from build123d import *

# Parameters (mm, degrees)
F0_W     = 50.0364415348
F0_H     = 37.788476795
F1_DEPTH = 81.28
F2_R     = 5.08
F3_T     = -2.54


# Not quite as in the source:
# - a shell that OpenCascade refuses in one call is made with other operations: the cavity is built on its own and cut out


with BuildPart() as f1:
    # F0 (on Front) → F1 (new body)
    with BuildSketch(Plane.XZ):
        with Locations((25.0182207674, -18.8942383975)):
            Rectangle(F0_W, F0_H)
    extrude(amount=F1_DEPTH)

    # F2
    f2_edges = [f1.edges().sort_by_distance(p)[0] for p in [
        (25.018221, -81.28, 0),
        (0, -81.28, -18.894238),
        (25.018221, -81.28, -37.788477),
        (50.036442, -81.28, -18.894238),
    ]]
    fillet(f2_edges, radius=F2_R)

    # F3: a shell. OpenCascade refuses it in one call, so the cavity is built on its own and cut out:
    # the body offset inwards by the wall thickness, plus a prism from it out through each open face.
    f3_core = offset(f1.part, amount=F3_T, mode=Mode.PRIVATE)
    f3_exits = [f3_core.faces().sort_by_distance(p)[0] for p in [
        (25.018221, -78.74, -18.894238),
    ]]
    add(f3_core, mode=Mode.SUBTRACT)
    extrude(f3_exits, amount=-F3_T, mode=Mode.SUBTRACT)


solid = f1.part
Could you check a few things on this model? Use its own coordinates, in mm. A direction names the side the tool comes from. Give positions to 0.01 mm unless a question says otherwise; leave off trailing zeros. Order: outer loops, then holes, each group sorted by start corner. A loop starts at its lowest first (then second) coordinate and runs counter-clockwise, first axis right, second up. Notation, with made-up numbers: (51, 10.25) - (66, 10.25) arc R6 ccw to (66, 16.25) - close; hole circle Ø9 at (51, 76). An arc over 180 degrees is marked (long way). Return JSON: item names as keys, results as strings. Group by question number.
Q1. Thinking about a two-plate mould opening in X: for faces 1 (the face through (25.37, -79.75, -36.34)), 2 (the face through (25.3, -78, -34.5)), 3 (the face through (25.333, -77.976, -3.264)), 4 (the face through (0, -38, -19)), which applies, pulls with the +X half, pulls with the -X half, needs draft (parallel to the pull), parting line crosses it, or undercut?
Q2. Which directions (+Z, -Z, +X, -X, +Y, -Y) give clear straight access to the entire face, cutting with the end or side of a thin tool? Please do faces 5 (the face through (25, -39, -2.54)), 6 (the face through (25, -80, -5.08)), 7 (the face through (25, -38, 0)).
Q3. Please list where these lines run through material, in increasing order: line 1 along X through (y, z) = (-54, -7.5); line 2 along Z through (x, y) = (16, -9.5); line 3 along Y through (x, z) = (4, -20). Write a range as [from, to].
Q4. Suppose I cut it at B-B, the plane z = -29. Please give me the cut outline in (x, y), and give its area (3 significant figures).
Q5. Will these pins go through, and if not, where does the flat tip stop? pin 1 Ø1.5 at (x, z) = (11.5, -20) entering from +Y; pin 2 Ø0.8 at (x, y) = (31, -79.5) entering from +Z; pin 3 Ø0.8 at (x, y) = (20.5, -80.5) entering from -Z; pin 4 Ø4 at (x, z) = (18, -15.5) entering from -Y.
Q6. Suppose I cut it at A-A, the plane y = -55.5. Please give me the cut outline in (x, z).
Q7. Suppose I cut it at C-C, the plane x = 12. Please give me the cut outline in (y, z), and give its area (3 significant figures).
Resolved:
{
 "1": {"face 1": "needs draft", "face 2": "undercut", "face 3": "undercut", "face 4": "pulls with the -X half"},
 "2": {"face 5": "none", "face 6": "-Y", "face 7": "+Z, +X, -X, +Y, -Y"},
 "3": {"line 1": "x = [0, 2.54], [47.5, 50.04]", "line 2": "z = [-37.79, -35.25], [-2.54, 0]", "line 3": "y = [-81.16, -78.5], [-2.54, 0]"},
 "4": {"outline": "(0, -76.2) arc R5.08 ccw to (5.08, -81.28) - (5.08, -78.74) arc R2.54 cw to (2.54, -76.2) - (2.54, -2.54) - (47.5, -2.54) - (47.5, -76.2) arc R2.54 cw to (44.96, -78.74) - (44.96, -81.28) arc R5.08 ccw to (50.04, -76.2) - (50.04, 0) - (0, 0) - close", "area": "532 mm2"},
 "5": {"pin 1": "stops at y = 0", "pin 2": "stops at z = -0.91", "pin 3": "stops at z = -35.96", "pin 4": "stops at y = -2.54"},
 "6": {"outline": "(0, -37.79) - (50.04, -37.79) - (50.04, 0) - (0, 0) - close; hole (2.54, -35.25) - (47.5, -35.25) - (47.5, -2.54) - (2.54, -2.54) - close"},
 "7": {"outline": "(-81.28, -32.71) arc R5.08 ccw to (-76.2, -37.79) - (0, -37.79) - (0, 0) - (-76.2, 0) arc R5.08 ccw to (-81.28, -5.08) - (-78.74, -5.08) arc R2.54 cw to (-76.2, -2.54) - (-2.54, -2.54) - (-2.54, -35.25) - (-76.2, -35.25) arc R2.54 cw to (-78.74, -32.71) - close", "area": "501 mm2"}
}
